from build123d import *

# Parameters (mm, degrees)
F0_W     = 38.4564194828
F0_H     = 33.5525823757
F1_DEPTH = 25.4
F2_W     = 60.9108451754
F2_H     = 5.1619354635


with BuildPart() as f1:
    # F0 (on Top) → F1 (new body, symmetric)
    with BuildSketch(Plane.XY):
        with Locations((0.3871461377, 2.0647742786)):
            Rectangle(F0_W, F0_H)
    extrude(amount=F1_DEPTH, both=True)

    # F2 (on Top) → F3 (revolve)
    with BuildSketch(Plane.XY):
        with Locations((-0.2580946311, 2.5809677318)):
            Rectangle(F2_W, F2_H)
    revolve(axis=Axis((-0.2580946311, 0, 0), (1, 0, 0)))


solid = f1.part
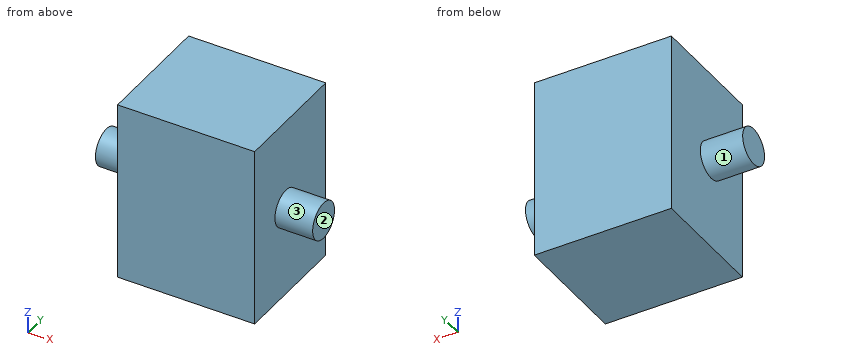
Verification items for the finished model (mm, model axes). Face numbers are marked on the shaded views. A direction names the side the tool comes from. Round coordinates to 2 decimals unless told otherwise and drop trailing zeros. Loops run counter-clockwise (first coordinate to the right, second up) from the corner with the lowest first, then second, coordinate; pieces in that order, holes last. Notation, with made-up numbers: (66, -32) - (86, -32) arc R22 ccw to (86, 3) - close; hole circle Ø6 at (-16.5, 19). An arc over 180 degrees is marked (long way). Use a Markdown table: item, result. Add a question column.
1. Gauge pin test, flat ends, axial feed: pin 1 (5 mm diameter, centred on y = -8.5, z = 14.5, fed in from -X); pin 2 (5 mm diameter, centred on x = -24.5, y = 6.5, fed in from +Z); pin 3 (2 mm diameter, centred on y = -1.5, z = -18.5, fed in from +X). Record the tip position at first contact, or that the pin passes through.
2. Section check D-D, the plane z = 14. Record the boundary of the cut face in (x, y).
3. Thickness scan on probe 1 along X at (y, z) = (12.5, -5). Record the ranges inside material, lowest first. Write a range as [from, to].
4. Access from +Z, -Z, +X, -X, +Y, -Y to the whole of each face (thin tool, end or side, straight path). Record for the marked faces 1, 2 and 3.
5. Section check B-B, the plane z = 0. Record the boundary of the cut face in (x, y).
6. Section check A-A, the plane y = 0. Record the boundary of the cut face in (x, z), plus the area to 3 significant figures.
7. Section check C-C, the plane x = 24.5. Record the boundary of the cut face in (y, z), plus the area to 3 significant figures.
Checks:
| question | item | result |
|---|---|---|
| 1 | pin 1 | stops at x = -18.84 |
| 1 | pin 2 | stops at z = 3.26 |
| 1 | pin 3 | stops at x = 19.62 |
| 2 | outline | (-18.84, -14.71) - (19.62, -14.71) - (19.62, 18.84) - (-18.84, 18.84) - close |
| 3 | probe 1 | x = [-18.84, 19.62] |
| 4 | face 1 | -X |
| 4 | face 2 | +Z, -Z, +X, +Y, -Y |
| 4 | face 3 | +X |
| 5 | outline | (-30.71, -5.16) - (-18.84, -5.16) - (-18.84, -14.71) - (19.62, -14.71) - (19.62, -5.16) - (30.2, -5.16) - (30.2, 5.16) - (19.62, 5.16) - (19.62, 18.84) - (-18.84, 18.84) - (-18.84, 5.16) - (-30.71, 5.16) - close |
| 6 | outline | (-30.71, -5.16) - (-18.84, -5.16) - (-18.84, -25.4) - (19.62, -25.4) - (19.62, -5.16) - (30.2, -5.16) - (30.2, 5.16) - (19.62, 5.16) - (19.62, 25.4) - (-18.84, 25.4) - (-18.84, 5.16) - (-30.71, 5.16) - close |
| 6 | area | 2,190 mm^2 |
| 7 | outline | circle Ø10.32 at (0, 0) |
| 7 | area | 83.7 mm^2 |
